Autodesk Inventor part; units mm, degrees
ref_plane "YZ Plane" through (0, 0, 0) normal (1, 0, 0) x (0, 1, 0)
ref_plane "XZ Plane" through (0, 0, 0) normal (0, 1, 0) x (-1, 0, 0)
ref_plane "XY Plane" through (0, 0, 0) normal (0, 0, 1) x (1, 0, 0)
sketch "Sketch1" plane through (0, 0, 0) normal (0, 1, 0) x (-1, 0, 0)
  line L0 (0, 0) -> (25.4, 0)
  line L1 (25.4, 0) -> (25.4, -25.4)
  line L2 (25.4, -25.4) -> (0, -25.4)
  line L3 (0, -25.4) -> (0, 0)
  line L4 (23.8125, -23.8125) -> (23.8125, -1.5875)
  line L5 (23.8125, -1.5875) -> (1.5875, -1.5875)
  line L6 (1.5875, -1.5875) -> (1.5875, -23.8125)
  line L7 (1.5875, -23.8125) -> (23.8125, -23.8125)
  dimension "d0" = 25.4
  dimension "d1" = 25.4
  dimension "d2" = 1.5875
extrude "Extrusion1" add sketch "Sketch1" along normal blind 736.6
sketch "Sketch2" plane through (-25.4, 0, 0) normal (0, 0, 1) x (1, 0, 0)
  circle A0 centre (12.7, 723.9) radius 6.35
  line L0 (0, 736.6) -> (25.4, 736.6)
  circle A1 centre (12.0929, 388.62) radius 6.35
  line L1 (0, 0) -> (0, 736.6)
  point P0 (25.4, 0)
  dimension "d5" = 12.7
  dimension "d6" = 12.7
  dimension "d7" = 12.7
  dimension "d8" = 347.98
  dimension "d11" = 12.0929
extrude "Extrusion2" cut sketch "Sketch2" against normal blind 25.4
sketch "Sketch3" plane through (0, 0, -25.4) normal (0, 0, -1) x (-1, 0, 0)
  point P0 (0, 0)
sketch "Sketch4" plane through (0, 0, -25.4) normal (0, 0, -1) x (-1, 0, 0)
  circle A0 centre (7.9502, 54.8132) radius 3.175
  line L0 (0, 0) -> (0, 736.6)
  line L1 (25.4, 0) -> (0, 0)
  dimension "d12" = 7.9502
  dimension "d13" = 54.8132
  dimension "d14" = 6.35
extrude "Extrusion3" cut sketch "Sketch4" against normal blind 25.4
properties part number "AP 1"
Work out the finished part from the listing and answer in its coordinate system (mm). A direction names the side the tool comes from. Give positions to 0.01 mm unless a question says otherwise; leave off trailing zeros. Order: outer loops, then holes, each group sorted by start corner. A loop starts at its lowest first (then second) coordinate and runs counter-clockwise, first axis right, second up.
1. The mould has two halves that part along Y. Classify faces 3 (the cylindrical face through (-14.134, 394.916, -0.783)), 4 (the flat face through (-1, 0, -13)), 5 (the flat face through (-1.588, 363, -13)): released by +Y, released by -Y, zero draft, split by the parting line, or undercut.
Result sheet:
face 3: undercut
face 4: released by -Y
face 5: zero draft
2. For faces 1 (the flat face through (-13, 363, -23.812)), 2 (the flat face through (-13, 363, 0)), determine the directions among +Z, -Z, +X, -X, +Y, -Y from which every point of the face is accessible in a straight line to the end or side of a thin tool.
Result sheet:
face 1: +Y, -Y
face 2: +Z, +X, -X, +Y, -Y
3. Straight lines are drawn through the part: L1, parallel to Y at x = -12.7, z = -0.6; L2, parallel to X at y = 37.5, z = -15.25. For each, find the intervals that lie inside material, in ascending order.
Result sheet:
L1: y = 0 to 382.3, 394.94 to 717.55, 730.25 to 736.6
L2: x = -25.4 to -23.81, -1.59 to 0
4. This flat-tipped pin is pushed along its axis until it touches: P1, Ø4, axis at x = -20.5, z = -19, coming from the -Y side. Where does it stop, or does it pass through?
Result sheet:
P1: passes through
5. Section C-C, the plane y = 388.62 is taken. Determine the outline of the cut face in (x, z), and give its area (3 significant figures).
Result sheet:
outline: (-25.4, -25.4) - (-19.66, -25.4) - (-19.66, -23.81) - (-23.81, -23.81) - (-23.81, -1.59) - (-19.66, -1.59) - (-19.66, 0) - (-25.4, 0) - close; (-6.96, -25.4) - (0, -25.4) - (0, 0) - (-6.96, 0) - (-6.96, -1.59) - (-1.59, -1.59) - (-1.59, -23.81) - (-6.96, -23.81) - close
area: 111 mm2
6. Section B-B, the plane z = -6.25 is taken. Determine the outline of the cut face in (x, y), and give its area (3 significant figures).
Result sheet:
outline: (-25.4, 0) - (-23.81, 0) - (-23.81, 736.6) - (-25.4, 736.6) - close; (-1.59, 0) - (0, 0) - (0, 736.6) - (-1.59, 736.6) - close
area: 2,340 mm2
7. Section A-A, the plane y = 560.5 is taken. Determine the outline of the cut face in (x, z).
Result sheet:
outline: (-25.4, -25.4) - (0, -25.4) - (0, 0) - (-25.4, 0) - close; hole (-23.81, -23.81) - (-1.59, -23.81) - (-1.59, -1.59) - (-23.81, -1.59) - close
